from build123d import *

# Parameters (mm, degrees)
SKETCH080_R           = 2.25
EXTRUDE081_DEPTH      = 0.6
EXTRUDE081_DEPTH_BACK = 2.4
SKETCH081_R           = 3.4
EXTRUDE080_DEPTH      = 2.4
EXTRUDE079_DEPTH      = 1.2
SKETCH075_R           = 1.8
SKETCH075_R_2         = 2.8
SKETCH075_R_3         = 3
EXTRUDE078_DEPTH      = 2


with BuildPart() as extrude081:
    # Sketch080 → Extrude081 (new body, two sides)
    with BuildSketch(Plane.XZ) as extrude081_sk:
        with Locations((-18.6, 12.1)):
            Circle(SKETCH080_R)
        with Locations((-18.6, 30.3)):
            Circle(SKETCH080_R)
        with Locations((-43.2, 30.3)):
            Circle(SKETCH080_R)
        with Locations((-43.2, 12.1)):
            Circle(SKETCH080_R)
    extrude(amount=EXTRUDE081_DEPTH)
    extrude(extrude081_sk.sketch, amount=-EXTRUDE081_DEPTH_BACK)


with BuildPart() as extrude080:
    # Sketch081 → Extrude080 (new body)
    with BuildSketch(Plane.XZ):
        with Locations((-43.2, 30.3)):
            Circle(SKETCH081_R)
        with Locations((-18.6, 30.3)):
            Circle(SKETCH081_R)
        with Locations((-43.2, 12.1)):
            Circle(SKETCH081_R)
        with Locations((-18.6, 12.1)):
            Circle(SKETCH081_R)
    extrude(amount=-EXTRUDE080_DEPTH)


with BuildPart() as obj1:
    # Sketch077 → Extrude079 (new body)
    with BuildSketch(Plane.XZ):
        with BuildLine():
            Line((-27.2, 26.7), (-27.2, 15.7))
            ThreePointArc((-27.2, 15.7), (-24.2, 12.7), (-21.2, 15.7))
            Line((-21.2, 26.700018), (-21.2, 15.7))
            ThreePointArc((-21.2, 26.700018), (-24.200009, 29.7), (-27.2, 26.7))
        make_face()
    extrude(amount=EXTRUDE079_DEPTH)


with BuildPart() as cut046:
    # Sketch075 → Extrude078 (new body)
    with BuildSketch(Plane.XZ):
        with BuildLine():
            Line((-82.8, 3.2), (0, 3.2))
            Line((0, 3.2), (0, 39.2))
            Line((-195.886839, 39.2), (0, 39.2))
            Line((-202.764796, 20.302968), (-195.886839, 39.2))
            ThreePointArc((-192.175575, -3.18451), (-192.085048, 10.987093), (-202.764796, 20.302968))
            Line((-192.175575, -3.18451), (-215.419579, -53.031439))
            ThreePointArc((-215.419579, -53.031439), (-218.578907, -66.677212), (-215.93199, -80.431568))
            Line((-215.93199, -80.431568), (-176.68528, -80.431568))
            Line((-147.645309, 8.944272), (-176.68528, -80.431568))
            ThreePointArc((-132.428405, 20), (-141.832969, 16.944272), (-147.645309, 8.944272))
            Line((-132.428405, 20), (-107.6, 20))
            ThreePointArc((-91.751972, 6.2), (-97.09286, 16.066483), (-107.6, 20))
            Line((-82.8, 6.2), (-91.751972, 6.2))
            Line((-82.8, 3.2), (-82.8, 6.2))
        make_face()
        with Locations((-213.443268, -76.831568)):
            Circle(SKETCH075_R, mode=Mode.SUBTRACT)
        with Locations((-179.304663, -76.831568)):
            Circle(SKETCH075_R, mode=Mode.SUBTRACT)
        with Locations((-184.079668, 34.8)):
            Circle(SKETCH075_R, mode=Mode.SUBTRACT)
        with Locations((-78.51, 34.8)):
            Circle(SKETCH075_R, mode=Mode.SUBTRACT)
        with Locations((-78.51, 7.6)):
            Circle(SKETCH075_R, mode=Mode.SUBTRACT)
        with Locations((-5.6, 34.8)):
            Circle(SKETCH075_R, mode=Mode.SUBTRACT)
        with Locations((-5.6, 7.6)):
            Circle(SKETCH075_R, mode=Mode.SUBTRACT)
        with Locations((-36.2, 21.2)):
            Circle(SKETCH075_R_2, mode=Mode.SUBTRACT)
        with Locations((-24.2, 26.7)):
            Circle(SKETCH075_R_3, mode=Mode.SUBTRACT)
        with Locations((-24.2, 15.7)):
            Circle(SKETCH075_R_3, mode=Mode.SUBTRACT)
        Polygon((-189.938695, 31.567195), (-192.332836, 24.989347), (-196.467483, 26.494236), (-194.073342, 33.072084), (-193.885404, 33.00368), (-190.126633, 31.635599), align=None, mode=Mode.SUBTRACT)
    extrude(amount=EXTRUDE078_DEPTH)

    # Cut045: cut obj1
    add(obj1.part, mode=Mode.SUBTRACT)

    # Fusion004: union Extrude080
    add(extrude080.part)

    # Cut046: cut Extrude081
    add(extrude081.part, mode=Mode.SUBTRACT)


solid = cut046.part
Can you work these out from the model? Positions are in its coordinate system, mm. A direction names the side the tool comes from. Give positions to 0.01 mm unless a question says otherwise; leave off trailing zeros. Loops run counter-clockwise (first coordinate to the right, second up) from the corner with the lowest first, then second, coordinate; pieces in that order, holes last. Notation, with made-up numbers: (-32.75, -20) - (2.25, -20) arc R25 ccw to (2.25, 7) - close; hole circle Ø7 at (-12.75, -1). An arc over 180 degrees is marked (long way). Return JSON: item names as keys, results as strings.
1. I want a section at A-A on y = 1.5. Please give me the cut outline in (x, z), and give its area (4 significant figures).
Output values:
{"outline": "circle Ø6.8 at (-43.2, 12.1); circle Ø6.8 at (-43.2, 30.3); circle Ø6.8 at (-18.6, 12.1); circle Ø6.8 at (-18.6, 30.3); hole circle Ø4.5 at (-43.2, 12.1); hole circle Ø4.5 at (-43.2, 30.3); hole circle Ø4.5 at (-18.6, 12.1); hole circle Ø4.5 at (-18.6, 30.3)", "area": "81.65 mm²"}
2. I want a section at B-B on x = -36.2. Please give me the cut outline in (y, z).
Output values:
{"outline": "(-2, 3.2) - (0, 3.2) - (0, 18.4) - (-2, 18.4) - close; (-2, 24) - (0, 24) - (0, 39.2) - (-2, 39.2) - close"}
3. For faces 1 (the face through (-22, 1.2, 30.4)), 2 (the face through (-16, 2.4, 30)), 3 (the face through (-141.719, -0.986, 17.026)), which set-ups out of +Z, -Z, +X, -X, +Y, -Y let a thin tool reach every point of the face, with its end or its side?
Output values:
{"face 1": "+Y", "face 2": "+Z, -Z, +X, -X, +Y", "face 3": "-Z, +Y, -Y"}
4. If I drill on line 1 (X direction, y = 0.8, z = 12); line 2 (Z direction, x = -43.2, y = 0.4); line 3 (Z direction, x = -78.51, y = -1), over which ranges is the centre line in solid material (lowest first)?
Output values:
{"line 1": "x = -46.6 to -45.45, -40.95 to -39.8, -22 to -20.85, -16.35 to -15.2", "line 2": "z = 8.7 to 9.85, 14.35 to 15.5, 26.9 to 28.05, 32.55 to 33.7", "line 3": "z = 3.2 to 5.8, 9.4 to 33, 36.6 to 39.2"}
5. I want a section at D-D on x = -103. Please give me the cut outline in (y, z).
Output values:
{"outline": "(-2, 19.32) - (0, 19.32) - (0, 39.2) - (-2, 39.2) - close"}
6. We'd pull the mould along X, two halves only. Please class faces 4 (the face through (-16, 2.4, 11)), 5 (the face through (-24.591, -1.208, 29.674)), 6 (the face through (-192, -1, 10.8)): +X half, -X half, draft (parallel to the pull), parting line (faces both ways), or undercut.
Output values:
{"face 4": "draft", "face 5": "undercut", "face 6": "-X half"}
7. I'm going to push flat-ended pins straight in: pin 1 Ø2 at (x, z) = (-44, 12.5) entering from +Y; pin 2 Ø0.6 at (x, y) = (-34.5, -1) entering from -Z; pin 3 Ø6 at (x, z) = (-78.51, 7.6) entering from +Y. Where does each tip first touch, or does it pass through?
Output values:
{"pin 1": "stops at y = -0.6", "pin 2": "stops at z = 3.2", "pin 3": "stops at y = 0"}
8. I want a section at C-C on z = -51. Please give me the cut outline in (x, y).
Output values:
{"outline": "(-214.47, -2) - (-167.12, -2) - (-167.12, 0) - (-214.47, 0) - close"}
